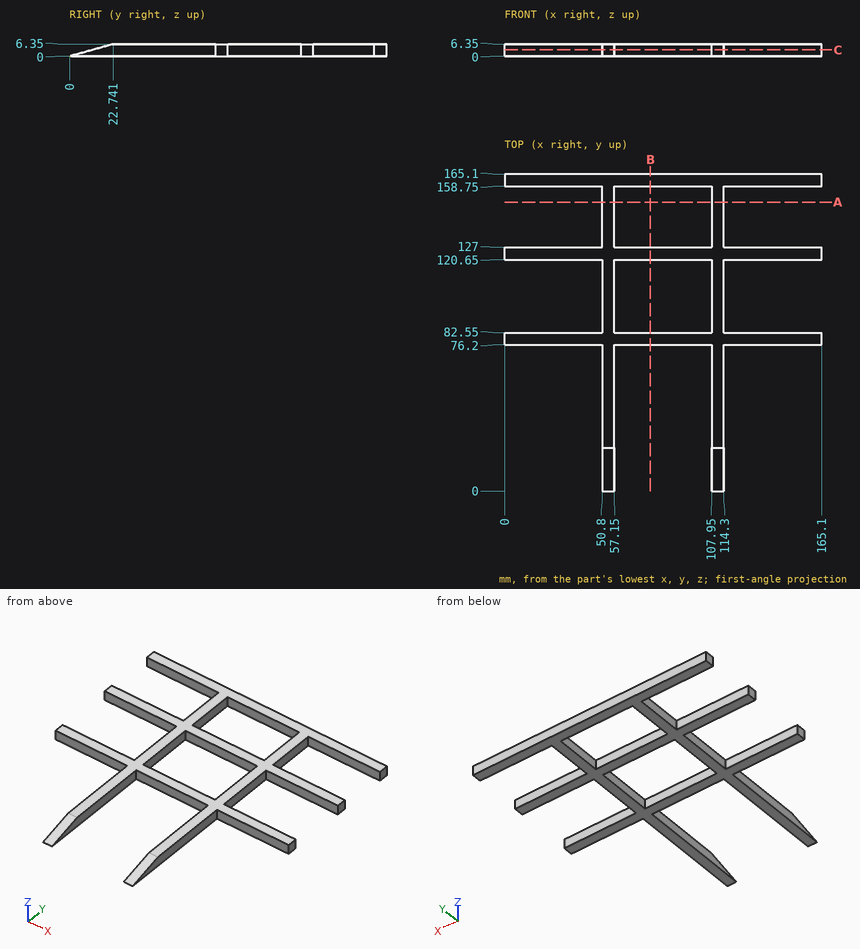
Verification items for this drawing (mm, ordinates from the low corner). Coordinates: 2 decimals unless noted, no trailing zeros. Loops run counter-clockwise (first coordinate to the right, second up) from the corner with the lowest first, then second, coordinate; pieces in that order, holes last. Notation, with made-up numbers: (25.5, 36) - (38.5, 36) arc R13 cw to (38.5, 60) - close; hole circle Ø10 at (85.25, -26). An arc over 180 degrees is marked (long way). Answer as a JSON object with one key per item and string values.
(1) Go/stop test with flat-tipped pins: pin 1 Ø3 at (x, z) = (95, 4.5) entering from -Y; pin 2 Ø1.9 at (y, z) = (96, 4) entering from +X. Record where each tip stops, or that it passes through.
Response:
{"pin 1": "stops at y = 76.2", "pin 2": "stops at x = 114.3"}
(2) Scan lines: line 1 along Y through (x, z) = (43.5, 2); line 2 along X through (y, z) = (118.5, 4.75). Record each from-to range of solid material in increasing order.
Response:
{"line 1": "y = 76.2 to 82.55, 120.65 to 127, 158.75 to 165.1", "line 2": "x = 50.8 to 57.15, 107.95 to 114.3"}
(3) Cross-section at C-C, the plane z = 3.25. Count the separate pieces of the cut face and the enclosed holes in it, then the cut area to 3 significant figures.
Response:
{"separate pieces": "1", "enclosed holes": "2", "area": "4,850 mm²"}
(4) Cross-section at B-B, the plane x = 76. Record the boundary of the cut face in (y, z).
Response:
{"outline": "(76.2, 0) - (82.55, 0) - (82.55, 6.35) - (76.2, 6.35) - close; (120.65, 0) - (127, 0) - (127, 6.35) - (120.65, 6.35) - close; (158.75, 0) - (165.1, 0) - (165.1, 6.35) - (158.75, 6.35) - close"}
(5) Cross-section at A-A, the plane y = 150.5. Record the boundary of the cut face in (x, z).
Response:
{"outline": "(50.8, 0) - (57.15, 0) - (57.15, 6.35) - (50.8, 6.35) - close; (107.95, 0) - (114.3, 0) - (114.3, 6.35) - (107.95, 6.35) - close"}
